The listing builds one solid part. Answer for the finished solid, in the listing's coordinates (mm). Face numbers are marked on the shaded views. A direction names the side the tool comes from. Coordinates: 2 decimals unless noted, no trailing zeros. Order: outer loops, then holes, each group sorted by start corner. A loop starts at its lowest first (then second) coordinate and runs counter-clockwise, first axis right, second up.
Autodesk Inventor part; units mm, degrees
ref_plane "YZ Plane" through (0, 0, 0) normal (1, 0, 0) x (0, 1, 0)
ref_plane "XZ Plane" through (0, 0, 0) normal (0, 1, 0) x (-1, 0, 0)
ref_plane "XY Plane" through (0, 0, 0) normal (0, 0, 1) x (1, 0, 0)
sketch "Sketch1" plane through (0, 0, 0) normal (1, 0, 0) x (0, 1, 0)
  circle A0 centre (0, 0) radius 11
  circle A1 centre (0, 0) radius 8.5
  dimension "d0" = 22
  dimension "d3" = 17
extrude "Extrusion1" add sketch "Sketch1" along normal blind 15
sketch "Sketch2" plane through (0, 0, 0) normal (0, 0, 1) x (1, 0, 0)
  line L0 (17.5, 2.5) -> (12.5, 2.5)
  line L1 (12.5, 2.5) -> (12.5, -2.5)
  line L2 (12.5, -2.5) -> (17.5, -2.5)
  line L3 (17.5, -2.5) -> (17.5, 2.5)
  line L4 (15, -11) -> (15, 11)
  line L5 (17.5, 2.5) -> (12.5, -2.5) construction
  line L6 (12.5, 2.5) -> (17.5, -2.5) construction
  circle A0 centre (12.5, 0) radius 2.5
  point P0 (0, 0)
  point P1 (15, 0)
  point P2 (15, -2.5)
  point P3 (15, 2.5)
  dimension "d4" = 5
  dimension "d5" = 5
extrude "Extrusion2" add sketch "Sketch2" along normal mid plane 34 contours L4 A0 L0 | A0 L1 | L1 A0 | L4 L2 A0
sketch "Sketch3" plane through (15, 0, 0) normal (1, 0, 0) x (0, 0, -1)
  circle A0 centre (0, 0) radius 9.5
  dimension "d8" = 19
extrude "Extrusion3" cut sketch "Sketch3" against normal blind 13.5
chamfer "Chamfer1" distance 1 angle 45 1 edges at (0, -11, 0)
sketch "Sketch4" plane through (0, 0, 0) normal (0, 1, 0) x (-1, 0, 0)
  line L0 (-15, 10.7121) -> (-15, -10.7121)
  circle A0 centre (-27, 0) radius 16.0857
  line L1 (-15, 0) -> (-27, 0) construction
  point P0 (0, 0)
  dimension "d14" = 12
extrude "Extrusion4" cut sketch "Sketch4" along normal through all both and the other way through all contours A0 L0 picked at (-13.6381, 0)
fillet "Fillet1" radius 2 2 edges at (15, 0, -10.7121) (15, 0, 10.7121)
properties part number "Cup" material "Aluminum 6061"
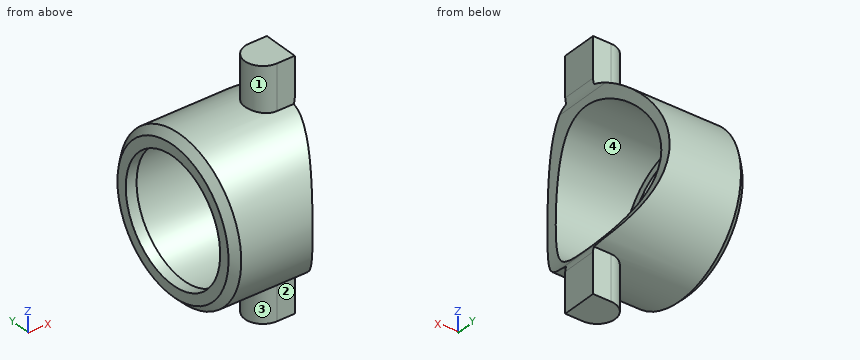
(1) Find section B-B (y = 0). Write down the section's boundary in (x, z), and give its area (3 significant figures).
(2) For the marked faces 1, 2, 3 and 4, determine the directions among +Z, -Z, +X, -X, +Y, -Y from which every point of the face is accessible in a straight line to the end or side of a thin tool.
(3) Find section A-A (z = 0). Write down the section's boundary in (x, y).
(4) Consider line 1 (Y direction, x = 1.15, z = 0); line 2 (Z direction, x = 9.75, y = 0); line 3 (Z direction, x = 8.25, y = 1). Determine where each line is inside the solid, lowest interval first.
(5) Find section D-D (z = -13.5). Write down the section's boundary in (x, y).
(6) Each of these flat-tipped pins is pushed along its axis until it touches: pin 1 Ø2 at (x, z) = (13.5, 13) entering from +Y; pin 2 Ø3 at (x, y) = (7.5, -7) entering from -Z; pin 3 Ø1.5 at (x, y) = (8, 2) entering from -Z. Where does it stop, or does it pass through?
(7) Find section C-C (x = 11.75). Write down the section's boundary in (y, z).
Findings below:
1. outline: (0, -10) - (1, -11) - (10, -11) - (10, -17) - (15, -17) - (15, -11.45) arc R2 ccw to (14.55, -10.18) arc R16.09 cw to (14.02, -9.5) - (1.5, -9.5) - (1.5, -8.5) - (0, -8.5) - close; (0, 8.5) - (1.5, 8.5) - (1.5, 9.5) - (14.02, 9.5) arc R16.09 cw to (14.55, 10.18) arc R2 ccw to (15, 11.45) - (15, 17) - (10, 17) - (10, 11) - (1, 11) - (0, 10) - close
1. area: 106 mm2
2. face 1: +Z, -X
2. face 2: -Z, +X, -X, -Y
2. face 3: -Z, -X
2. face 4: +X
3. outline: (0, -10) - (1, -11) - (10.91, -11) - (10.91, -9.5) - (1.5, -9.5) - (1.5, -8.5) - (0, -8.5) - close; (0, 8.5) - (1.5, 8.5) - (1.5, 9.5) - (10.91, 9.5) - (10.91, 11) - (1, 11) - (0, 10) - close
4. line 1: y = -11 to -8.5, 8.5 to 11
4. line 2: z = -11 to -9.5, 9.5 to 11
4. line 3: z = -10.95 to -9.45, 9.45 to 10.95
5. outline: (12.5, -2.5) - (15, -2.5) - (15, 2.5) - (12.5, 2.5) arc R2.5 ccw to start
6. pin 1: stops at y = 2.5
6. pin 2: stops at z = -9.53
6. pin 3: stops at z = -10.93
7. outline: (-9.74, -5.12) arc R11 ccw to (-2.38, -10.74) - (-2.38, -17) - (2.38, -17) - (2.38, -10.74) arc R11 ccw to (9.74, -5.12) - (8, -5.12) arc R9.5 cw to (-8, -5.12) - close; (-9.74, 5.12) - (-8, 5.12) arc R9.5 cw to (8, 5.12) - (9.74, 5.12) arc R11 ccw to (2.38, 10.74) - (2.38, 17) - (-2.38, 17) - (-2.38, 10.74) arc R11 ccw to start
